from build123d import *

# Parameters (mm, degrees)
BOSS_EXTRUDE1_DEPTH = 1003.3
BOSS_EXTRUDE2_DEPTH = 25.4
SKETCH3_W           = 101.6
SKETCH3_H           = 19.05
CUT_EXTRUDE1_DEPTH  = 7.35
SKETCH4_R           = 3.175
CUT_EXTRUDE2_DEPTH  = 756.65
SKETCH5_W           = 31.75
SKETCH5_H           = 38.1
CUT_EXTRUDE3_DEPTH  = 6.35


with BuildPart() as part:
    # Sketch1 → Boss-Extrude1 (new body)
    with BuildSketch(Plane(origin=(0, 0, 0), x_dir=(0, 0, -1), z_dir=(1, 0, 0))):
        Polygon((0, 0), (0, 31.75), (-6.35, 31.75), (-6.35, -6.35), (31.75, -6.35), (31.75, 0), align=None)
    extrude(amount=BOSS_EXTRUDE1_DEPTH)

    # Sketch2 → Boss-Extrude2 (add)
    with BuildSketch(Plane(origin=(0, 0, 0), x_dir=(1, 0, 0), z_dir=(0, 1, 0))):
        Polygon((247.65, 31.75), (254, 31.75), (254, 0), (222.25, 0), (222.25, 6.35), (247.65, 6.35), align=None)
        Polygon((387.35, 6.35), (387.35, 0), (355.6, 0), (355.6, 31.75), (361.95, 31.75), (361.95, 6.35), align=None)
    extrude(amount=BOSS_EXTRUDE2_DEPTH)

    # Sketch3 → Cut-Extrude1 (cut, through all)
    with BuildSketch(Plane(origin=(0, 0, 0), x_dir=(1, 0, 0), z_dir=(0, 1, 0))):
        with Locations((304.8, 22.225)):
            Rectangle(SKETCH3_W, SKETCH3_H)
    extrude(amount=-CUT_EXTRUDE1_DEPTH, mode=Mode.SUBTRACT)

    # Sketch4 → Cut-Extrude2 (cut, through all)
    with BuildSketch(Plane.ZY.offset(-247.65)):
        with Locations((-19.05, 9.525)):
            Circle(SKETCH4_R)
    extrude(amount=-CUT_EXTRUDE2_DEPTH, mode=Mode.SUBTRACT)

    # Sketch5 → Cut-Extrude3 (cut)
    with BuildSketch(Plane.XY.offset(6.35)):
        with Locations((15.875, 12.7)):
            Rectangle(SKETCH5_W, SKETCH5_H)
        with Locations((987.425, 12.7)):
            Rectangle(SKETCH5_W, SKETCH5_H)
    extrude(amount=-CUT_EXTRUDE3_DEPTH, mode=Mode.SUBTRACT)


solid = part.part
Model file for the job. Use its own axes, mm. A direction names the side the tool comes from. Give positions to 0.01 mm unless a question says otherwise; leave off trailing zeros. Order: outer loops, then holes, each group sorted by start corner. A loop starts at its lowest first (then second) coordinate and runs counter-clockwise, first axis right, second up. Notation, with made-up numbers: (13.5, -1) - (38.5, -1) arc R11 ccw to (38.5, 16) - close; hole circle Ø4 at (-38.75, -7). An arc over 180 degrees is marked (long way). One line per item, written item: value.
Item 1: Pin check, flat tips, straight feed: pin 1 Ø5 at (y, z) = (19.5, 4.5) entering from -X; pin 2 Ø16 at (x, z) = (371, -20) entering from +Y; pin 3 Ø9.5 at (x, y) = (719, 14.5) entering from -Z; pin 4 Ø5.5 at (y, z) = (9.525, -19.05) entering from +X. Stop position of each tip, or through.
Response values:
pin 1: x = 31.75
pin 2: y = 0
pin 3: z = 0
pin 4: through
Item 2: Slice it at A-A (x = 396). List the corners of the cut face in (y, z).
Response values:
outline: (-6.35, -31.75) - (0, -31.75) - (0, 0) - (31.75, 0) - (31.75, 6.35) - (-6.35, 6.35) - close
Item 3: Tool access for faces 1 (the flat face through (235, 13, -6.35)), 2 (the flat face through (365, 25.4, -6)), 3 (the flat face through (495, 16, 0)): list every direction of +Z, -Z, +X, -X, +Y, -Y with a clear straight run to the whole face (end or side of a thin tool).
Response values:
face 1: -Z, -X, +Y
face 2: -Z, +X, -X, +Y
face 3: -Z, +Y
Item 4: Two-plate mould, pull along X, no slides. Class faces 4 (the flat face through (254, 13, -16)), 5 (the flat face through (247.65, 15, -19)), 6 (the flat face through (374, 13, -6.35)): released by +X, released by -X, zero draft, split by the parting line, or undercut.
Response values:
face 4: undercut
face 5: released by -X
face 6: zero draft
Item 5: Wall check: line 1 (X direction, y = 14, z = -26); line 2 (Y direction, x = 249, z = -19); line 3 (X direction, y = 12.5, z = 1.5). Give the ranges that are in metal, low to high.
Response values:
line 1: 247.65 to 254, 355.6 to 361.95
line 2: -6.35 to 6.35, 12.7 to 25.4
line 3: 31.75 to 971.55
